from build123d import *

# Parameters (mm, degrees)
SKETCH1_W           = 54.864
SKETCH1_H           = 280.162
SKETCH1_W_2         = 3.683
SKETCH1_H_2         = 260.604
BOSS_EXTRUDE1_DEPTH = 3.175
SKETCH2_W           = 3.175
SKETCH2_H           = 101.6
BOSS_EXTRUDE2_DEPTH = 3.175
SKETCH3_W           = 225.425
SKETCH3_H           = 6.35
BOSS_EXTRUDE3_DEPTH = 51.689
SKETCH7_W           = 327.022738736
SKETCH7_H           = 279.435650021
CUT_EXTRUDE1_DEPTH  = 55.864
SKETCH4_W           = 6.35
SKETCH4_H           = 3.175
SKETCH4_W_2         = 4.8895
SKETCH4_H_2         = 12.7
CUT_EXTRUDE2_DEPTH  = 6.35
SKETCH8_W           = 9.525
SKETCH8_H           = 25.4
BOSS_EXTRUDE4_DEPTH = 3.175
SKETCH9_W           = 3.175
SKETCH9_H           = 16.933333333
SKETCH9_H_2         = 16.933333334
CUT_EXTRUDE4_DEPTH  = 4.175
SKETCH10_W          = 6.35
SKETCH10_H          = 3.175
CUT_EXTRUDE5_DEPTH  = 4.175
SKETCH13_W          = 9.525
SKETCH13_H          = 11.43
CUT_EXTRUDE7_DEPTH  = 4.175
SKETCH14_R          = 3.81
CUT_EXTRUDE8_DEPTH  = 4.175
FILLET1_R           = 2.54


with BuildPart() as part:
    # Sketch1 → Boss-Extrude1 (new body)
    with BuildSketch(Plane.XY):
        with Locations((0, 3.429)):
            Rectangle(SKETCH1_W, SKETCH1_H)
        Rectangle(SKETCH1_W_2, SKETCH1_H_2, mode=Mode.SUBTRACT)
    extrude(amount=BOSS_EXTRUDE1_DEPTH)

    # Sketch2 → Boss-Extrude2 (add)
    with BuildSketch(Plane(origin=(27.432, 0, 0), x_dir=(0, 0, -1), z_dir=(1, 0, 0))):
        Polygon((225.425, -47.752), (225.425, -35.052), (0, -35.052), (0, -136.652), (225.425, -136.652), (225.425, -123.952), (228.6, -123.952), (228.6, -107.018666667), (225.425, -107.018666667), (225.425, -94.318666667), (228.6, -94.318666667), (228.6, -77.385333333), (225.425, -77.385333333), (225.425, -64.685333333), (228.6, -64.685333333), (228.6, -47.752), align=None)
        with BuildLine():
            ThreePointArc((11.4, -103.892), (9.9, -105.392), (8.4, -103.892))
            Line((8.4, -103.892), (8.4, -98.812))
            ThreePointArc((8.4, -98.812), (9.9, -97.312), (11.4, -98.812))
            Line((11.4, -98.812), (11.4, -103.892))
        make_face(mode=Mode.SUBTRACT)
        with BuildLine():
            Line((42.4, -98.812), (42.4, -103.892))
            ThreePointArc((42.4, -103.892), (40.9, -105.392), (39.4, -103.892))
            Line((39.4, -103.892), (39.4, -98.812))
            ThreePointArc((39.4, -98.812), (40.9, -97.312), (42.4, -98.812))
        make_face(mode=Mode.SUBTRACT)
        with BuildLine():
            ThreePointArc((36.4, -88.392), (25.4, -99.392), (14.4, -88.392))
            Line((14.4, -88.392), (14.4, -83.312))
            ThreePointArc((14.4, -83.312), (25.4, -72.312), (36.4, -83.312))
            Line((36.4, -83.312), (36.4, -88.392))
        make_face(mode=Mode.SUBTRACT)
        with BuildLine():
            ThreePointArc((11.4, -72.892), (9.9, -74.392), (8.4, -72.892))
            Line((8.4, -72.892), (8.4, -67.812))
            ThreePointArc((8.4, -67.812), (9.9, -66.312), (11.4, -67.812))
            Line((11.4, -67.812), (11.4, -72.892))
        make_face(mode=Mode.SUBTRACT)
        with BuildLine():
            ThreePointArc((42.4, -72.892), (40.9, -74.392), (39.4, -72.892))
            Line((39.4, -72.892), (39.4, -67.812))
            ThreePointArc((39.4, -67.812), (40.9, -66.312), (42.4, -67.812))
            Line((42.4, -67.812), (42.4, -72.892))
        make_face(mode=Mode.SUBTRACT)
        with Locations((-1.5875, -85.852)):
            Rectangle(SKETCH2_W, SKETCH2_H)
    extrude(amount=-BOSS_EXTRUDE2_DEPTH)

    # Sketch3 → Boss-Extrude3 (add)
    with BuildSketch(Plane.ZY.offset(-24.257)):
        with Locations((-112.7125, -133.477)):
            Rectangle(SKETCH3_W, SKETCH3_H)
    extrude(amount=BOSS_EXTRUDE3_DEPTH)

    # Sketch7 → Cut-Extrude1 (cut, through all)
    with BuildSketch(Plane(origin=(27.432, 0, 0), x_dir=(0, 0, -1), z_dir=(1, 0, 0))):
        with Locations((163.511369368, -148.348068682)):
            Rectangle(SKETCH7_W, SKETCH7_H)
    extrude(amount=-CUT_EXTRUDE1_DEPTH, mode=Mode.SUBTRACT)

    # Sketch4 → Cut-Extrude2 (cut)
    with BuildSketch(Plane.XZ.offset(136.652)):
        with Locations((-12.8905, 1.5875)):
            Rectangle(SKETCH4_W, SKETCH4_H)
        with Locations((24.98725, 1.5875)):
            Rectangle(SKETCH4_W_2, SKETCH4_H)
        with Locations((-24.98725, 1.5875)):
            Rectangle(SKETCH4_W_2, SKETCH4_H)
        with Locations((12.8905, 1.5875)):
            Rectangle(SKETCH4_W, SKETCH4_H)
        with Locations((24.98725, -138.1125)):
            Rectangle(SKETCH4_W_2, SKETCH4_H_2)
        with Locations((24.98725, -57.15)):
            Rectangle(SKETCH4_W_2, SKETCH4_H_2)
        with Locations((24.98725, -165.1)):
            Rectangle(SKETCH4_W_2, SKETCH4_H_2)
    extrude(amount=-CUT_EXTRUDE2_DEPTH, mode=Mode.SUBTRACT)

    # Sketch8 → Boss-Extrude4 (add)
    with BuildSketch(Plane.XY.offset(3.175)):
        with Locations((-32.1945, 119.38)):
            Rectangle(SKETCH8_W, SKETCH8_H)
        with Locations((32.1945, 119.38)):
            Rectangle(SKETCH8_W, SKETCH8_H)
    extrude(amount=-BOSS_EXTRUDE4_DEPTH)

    # Sketch9 → Cut-Extrude4 (cut, through all)
    with BuildSketch(Plane.XY.offset(3.175)):
        with Locations((-10.4775, -56.218666666)):
            Rectangle(SKETCH9_W, SKETCH9_H)
        with Locations((-10.4775, -85.852)):
            Rectangle(SKETCH9_W, SKETCH9_H_2)
        with Locations((-10.4775, -115.485333334)):
            Rectangle(SKETCH9_W, SKETCH9_H)
        with Locations((10.4775, -56.218666666)):
            Rectangle(SKETCH9_W, SKETCH9_H)
        with Locations((10.4775, -85.852)):
            Rectangle(SKETCH9_W, SKETCH9_H_2)
        with Locations((10.4775, -115.485333334)):
            Rectangle(SKETCH9_W, SKETCH9_H)
    extrude(amount=-CUT_EXTRUDE4_DEPTH, mode=Mode.SUBTRACT)

    # Sketch10 → Cut-Extrude5 (cut, through all)
    with BuildSketch(Plane.XY.offset(3.175)):
        with Locations((0, 136.9695)):
            Rectangle(SKETCH10_W, SKETCH10_H)
    extrude(amount=-CUT_EXTRUDE5_DEPTH, mode=Mode.SUBTRACT)

    # Sketch13 → Cut-Extrude7 (cut, through all)
    with BuildSketch(Plane.XY.offset(3.175)):
        with Locations((0, -77.597)):
            Rectangle(SKETCH13_W, SKETCH13_H)
    extrude(amount=-CUT_EXTRUDE7_DEPTH, mode=Mode.SUBTRACT)

    # Sketch14 → Cut-Extrude8 (cut, through all)
    with BuildSketch(Plane.XY.offset(3.175)):
        with Locations((12.192, -23.3172)):
            Circle(SKETCH14_R)
    extrude(amount=-CUT_EXTRUDE8_DEPTH, mode=Mode.SUBTRACT)

    # Fillet1
    fillet1_edges = [part.edges().sort_by_distance(p)[0] for p in [
        (-1.8415, -83.312, 1.5875),
        (-1.8415, -71.882, 1.5875),
        (1.8415, -71.882, 1.5875),
        (1.8415, -83.312, 1.5875),
    ]]
    fillet(fillet1_edges, radius=FILLET1_R)


solid = part.part
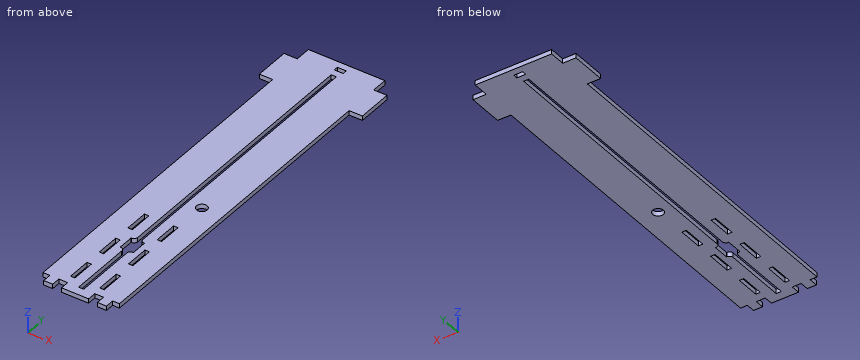
For this review, take the finished solid that the model builds, in its own axes (mm). Coordinates: 2 decimals unless noted, no trailing zeros. Loops run counter-clockwise (first coordinate to the right, second up) from the corner with the lowest first, then second, coordinate; pieces in that order, holes last. Notation, with made-up numbers: (-20.75, 59.25) - (-10.75, 59.25) arc R6 cw to (-10.75, 69.25) - close; hole circle Ø2 at (70, 0). An arc over 180 degrees is marked (long way). Use a Markdown table: item, result. Add a question column.
Item 1: Insertion check: pin 1 Ø1 at (y, z) = (137, 1) entering from -X; pin 2 Ø1 at (y, z) = (-58, 1.5) entering from +X; pin 3 Ø1 at (x, z) = (33.5, 1.5) entering from +Y. Each pin has a flat end and moves straight along its axis. Give the tip position at first contact, or say it passes through.
Item 2: We need section D-D (x = 25). Give the boundary of the cut face in (y, z) (3 decimals).
Item 3: We need section B-B (y = -112). Give the boundary of the cut face in (x, z) (1 decimal), and give its area (3 significant figures).
Item 4: We need section A-A (y = -3). Give the boundary of the cut face in (x, z) (1 decimal).
Item 5: For line 1 (X direction, y = -111, z = 1.9) (1 decimal); line 2 (X direction, y = -79, z = 0.9) (1 decimal); line 3 (X direction, y = 115.5, z = 2.75), list the stretches that pass through material, from the lowest coordinate up.
Item 6: We need section C-C (y = 113). Give the boundary of the cut face in (x, z) (1 decimal).
Results list:
| question | item | result |
|---|---|---|
| 1 | pin 1 | stops at x = -27.43 |
| 1 | pin 2 | stops at x = 27.43 |
| 1 | pin 3 | stops at y = 132.08 |
| 2 | outline | (-130.302, 0) - (143.51, 0) - (143.51, 3.175) - (-130.302, 3.175) - close |
| 3 | outline | (-27.4, 0) - (-12.1, 0) - (-12.1, 3.2) - (-27.4, 3.2) - close; (-8.9, 0) - (-1.8, 0) - (-1.8, 3.2) - (-8.9, 3.2) - close; (1.8, 0) - (8.9, 0) - (8.9, 3.2) - (1.8, 3.2) - close; (12.1, 0) - (27.4, 0) - (27.4, 3.2) - (12.1, 3.2) - close |
| 3 | area | 142 mm^2 |
| 4 | outline | (-27.4, 0) - (-1.8, 0) - (-1.8, 3.2) - (-27.4, 3.2) - close; (1.8, 0) - (27.4, 0) - (27.4, 3.2) - (1.8, 3.2) - close |
| 5 | line 1 | x = -27.4 to -12.1, -8.9 to -1.8, 1.8 to 8.9, 12.1 to 27.4 |
| 5 | line 2 | x = -27.4 to -12.1, -8.9 to -4.8, 4.8 to 8.9, 12.1 to 27.4 |
| 5 | line 3 | x = -36.96 to -1.84, 1.84 to 36.96 |
| 6 | outline | (-37, 0) - (-1.8, 0) - (-1.8, 3.2) - (-37, 3.2) - close; (1.8, 0) - (37, 0) - (37, 3.2) - (1.8, 3.2) - close |
